For this review, take the finished solid that the model builds, in its own axes (mm). A direction names the side the tool comes from. Round coordinates to 2 decimals unless told otherwise and drop trailing zeros. Write each loop counter-clockwise with the first axis right and the second up, starting at its lowest first coordinate (ties: lowest second). Pieces come first, ordered by that corner, then holes. Notation, with made-up numbers: (24.25, -39) -> (82.25, -39) arc R15 ccw to (82.25, -31) -> close; hole circle Ø8 at (8.5, 23.25). An arc over 180 degrees is marked (long way). Answer in a Markdown table with one row per item.
Autodesk Inventor part; units mm, degrees
ref_plane "Work Plane1" through (0, 15, 0) normal (0, 1, 0) x (-1, 0, 0)
ref_plane "YZ Plane" through (0, 0, 0) normal (1, 0, 0) x (0, 1, 0)
ref_plane "XY Plane" through (0, 0, 0) normal (0, 0, 1) x (1, 0, 0)
sketch "Sketch1" plane through (0, 0, 0) normal (0, 1, 0) x (-1, 0, 0)
  line L0 (-12.6, 0) -> (-15.4, 0)
  line L1 (0, -53.2) -> (0, 53.2)
  line L2 (-13, -38) -> (-15, -38)
  line L3 (-15, -38) -> (-15, 38)
  line L4 (-15, 38) -> (-13, 38)
  line L5 (-13, 38) -> (-13, -38)
  line L6 (-13, -38) -> (-15, 38) construction
  line L7 (-15, -38) -> (-13, 38) construction
  point P0 (-14, 0)
  dimension "d0" = 2
  dimension "d1" = 76
  dimension "d2" = 30
revolve "Revolution1" add sketch "Sketch1" angle 360 about axis through (0, 0, -10) along (0, 0, 1)
ref_plane "Work Plane1" through (0, 15, 0) normal (0, 1, 0) x (-1, 0, 0)
sketch "Sketch3" plane through (0, 15, 0) normal (0, 1, 0) x (-1, 0, 0)
  line L0 (-7.5, -20) -> (7.5, -20)
  line L1 (7.5, -20) -> (7.5, 20)
  line L2 (7.5, 20) -> (-7.5, 20)
  line L3 (-7.5, 20) -> (-7.5, -20)
  line L4 (-7.5, -20) -> (7.5, 20) construction
  line L5 (7.5, -20) -> (-7.5, 20) construction
  point P0 (0, 0)
  dimension "d4" = 15
  dimension "d5" = 40
extrude "Extrusion1" cut sketch "Sketch3" against normal blind 3
sketch "Sketch5" plane through (0, 0, -38) normal (0, 0, -1) x (-1, 0, 0)
  circle A0 centre (0, 0) radius 13
  circle A1 centre (0, 0) radius 16
  dimension "d8" = 32
  dimension "d9" = 26
extrude "Extrusion2" add sketch "Sketch5" along normal blind 8
sketch "Sketch6" plane through (0, 0, 38) normal (0, 0, 1) x (1, 0, 0)
  circle A0 centre (0, 0) radius 13
  circle A1 centre (0, 0) radius 16
  dimension "d12" = 26
  dimension "d13" = 32
extrude "Extrusion3" add sketch "Sketch6" along normal blind 6
properties part number "Handle bars holder axle"
1) For faces 4 (the flat face through (-6, 12, 0)), 5 (the cylindrical face through (3.47, 15.62, -41.94)), list the 3-axis set-ups (+Z, -Z, +X, -X, +Y, -Y) from which the entire face can be reached by the end or side of a thin tool; tool diameter is ignored.
Solved:
| item | result |
|---|---|
| face 4 | +Y |
| face 5 | +Z, -Z |
2) Consider section A-A on y = 0. State the section outline as (x, z) points.
Solved:
| item | result |
|---|---|
| outline | (-16, -46) -> (-13, -46) -> (-13, 44) -> (-16, 44) -> (-16, 38) -> (-15, 38) -> (-15, -38) -> (-16, -38) -> close; (13, -46) -> (16, -46) -> (16, -38) -> (15, -38) -> (15, 38) -> (16, 38) -> (16, 44) -> (13, 44) -> close |
3) Mouldability with a two-part tool opening along Z and no side actions: class faces 1 (the cylindrical face through (-3.47, 15.62, 40.96)), 2 (the flat face through (-1.3, 13.1, 44)), 3 (the cylindrical face through (-3.252, -14.643, 0.532)) as pulls with the +Z half, pulls with the -Z half, needs draft (parallel to the pull), parting line crosses it, or undercut.
Solved:
| item | result |
|---|---|
| face 1 | needs draft |
| face 2 | pulls with the +Z half |
| face 3 | undercut |
4) For line 1 (Y direction, x = 0, z = 39); line 2 (X direction, y = 4, z = -22); line 3 (Y direction, x = 0, z = 16), list the stretches that pass through material, from the lowest coordinate up. Write a range as [from, to].
Solved:
| item | result |
|---|---|
| line 1 | [-16, -13], [13, 16] |
| line 2 | [-14.46, -12.37], [12.37, 14.46] |
| line 3 | [-15, -13] |
5) Consider section B-B on x = 0. State the section outline as (y, z) points.
Solved:
| item | result |
|---|---|
| outline | (-16, -46) -> (-13, -46) -> (-13, 44) -> (-16, 44) -> (-16, 38) -> (-15, 38) -> (-15, -38) -> (-16, -38) -> close; (13, -46) -> (16, -46) -> (16, -38) -> (15, -38) -> (15, -20) -> (13, -20) -> close; (13, 20) -> (15, 20) -> (15, 38) -> (16, 38) -> (16, 44) -> (13, 44) -> close |
6) Consider section D-D on z = 25. State the section outline as (x, y) points.
Solved:
| item | result |
|---|---|
| outline | circle Ø30 at (0, 0); hole circle Ø26 at (0, 0) |
7) Clearance check with flat-ended pins moving along their axes: pin 1 Ø5 at (x, y) = (8, -1) entering from +Z; pin 2 Ø8 at (y, z) = (-10, -10) entering from -X; pin 3 Ø1 at (y, z) = (4, -23.5) entering from -X; pin 4 Ø10 at (y, z) = (-2, 8.5) entering from -X. State where each tip first meets the part, or that it passes through.
Solved:
| item | result |
|---|---|
| pin 1 | through |
| pin 2 | x = -13.75 |
| pin 3 | x = -14.59 |
| pin 4 | x = -15 |
8) Consider section C-C on z = 5. State the section outline as (x, y) points.
Solved:
| item | result |
|---|---|
| outline | (-7.5, 12) -> (-7.5, 12.99) arc R15 ccw (long way) to (7.5, 12.99) -> (7.5, 12) -> (5, 12) arc R13 cw (long way) to (-5, 12) -> close |
